Job drawing, mm, ordinate dimensions from the low corner. One solid piece. Round coordinates to 2 decimals unless told otherwise and drop trailing zeros. Write each loop counter-clockwise with the first axis right and the second up, starting at its lowest first coordinate (ties: lowest second). Pieces come first, ordered by that corner, then holes.
1) Drill centre lines: L1, parallel to Z at x = 17, y = 12.5; L2, parallel to X at y = 10.5, z = 235; L3, parallel to Y at x = 17.25, z = 18. Where is each one in solid material? Low to high.
2) Flat gauge pins, fed straight in: pin 1 (16 mm diameter, centred on x = 15, z = 234.5, fed in from -Y); pin 2 (10 mm diameter, centred on y = 7.5, z = 237.5, fed in from -X). Where does each tip first touch, or does it go through?
3) Saw through at A-A on x = 11.5. Write the cut outline in (y, z).
4) Saw through at B-B on y = 16. Write the cut outline in (x, z).
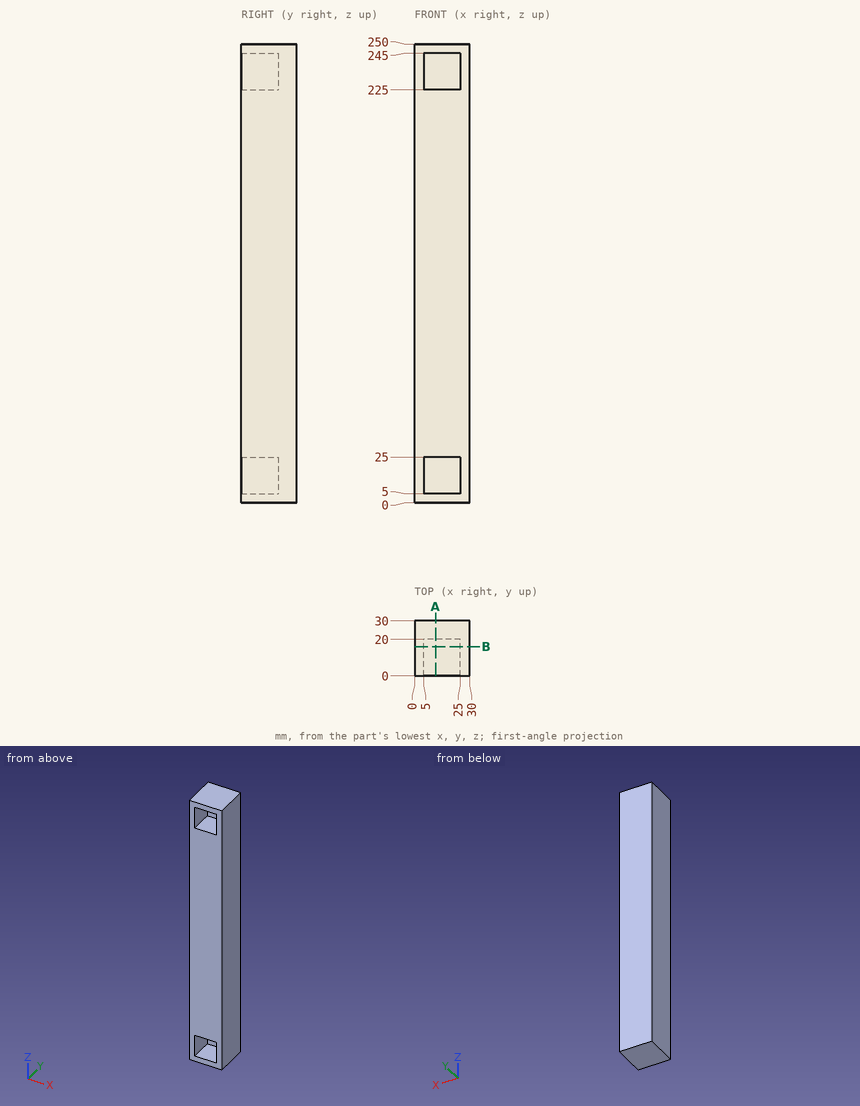
Completed:
1. L1: z = 0 to 5, 25 to 225, 245 to 250
1. L2: x = 0 to 5, 25 to 30
1. L3: y = 20 to 30
2. pin 1: stops at y = 20
2. pin 2: stops at x = 0
3. outline: (0, 0) - (30, 0) - (30, 250) - (0, 250) - (0, 245) - (20, 245) - (20, 225) - (0, 225) - (0, 25) - (20, 25) - (20, 5) - (0, 5) - close
4. outline: (0, 0) - (30, 0) - (30, 250) - (0, 250) - close; hole (5, 5) - (25, 5) - (25, 25) - (5, 25) - close; hole (5, 225) - (25, 225) - (25, 245) - (5, 245) - close
